```python
from build123d import *

# Parameters (mm, degrees)
CROQUIS1_W              = 30
CROQUIS1_H              = 49
SALIENTE_EXTRUIR1_DEPTH = 20
CORTAR_EXTRUIR3_DEPTH   = 20
CORTAR_EXTRUIR5_DEPTH   = 20
CORTAR_EXTRUIR6_DEPTH   = 0.3
CROQUIS5_W              = 13.233735145
CROQUIS5_H              = 2.403316153
CORTAR_EXTRUIR9_DEPTH   = 20.3
CROQUIS6_W              = 2.5
CROQUIS6_H              = 19.5
SALIENTE_EXTRUIR2_DEPTH = 29
REDONDEO1_R             = 9
CORTAR_EXTRUIR10_DEPTH  = 29
CORTAR_EXTRUIR11_DEPTH  = 29
CORTAR_EXTRUIR16_DEPTH  = 9
CORTAR_EXTRUIR17_START  = -2
CORTAR_EXTRUIR17_DEPTH  = 9
CROQUIS13_R             = 0.40141899
CORTAR_EXTRUIR18_DEPTH  = 22
MATRIZC1_COUNT          = 15
MATRIZC1_ANGLE          = 82


with BuildPart() as part:
    # Croquis1 → Saliente-Extruir1 (new body)
    with BuildSketch(Plane.XY):
        Rectangle(CROQUIS1_W, CROQUIS1_H)
    extrude(amount=SALIENTE_EXTRUIR1_DEPTH)

    # Croquis2 → Cortar-Extruir3 (cut)
    with BuildSketch(Plane.XY.offset(20)):
        with BuildLine():
            ThreePointArc((-0.474525342, 13.297985817), (-5.593414892, 15.404003131), (-9.517328589, 11.5))
            ThreePointArc((-9.517328589, 11.5), (-9.593029868, 11.00254481), (-9.618349103, 10.5))
            ThreePointArc((-9.618349103, 10.5), (-9.39256168, 9.014438062), (-8.735591395, 7.663044605))
            ThreePointArc((-8.735591395, 7.663044605), (-8.404944841, 7.234775243), (-8.029958496, 6.84474059))
            ThreePointArc((-8.029958496, 6.84474059), (-5.140673383, 3.522596276), (-3, -0.324757201))
            ThreePointArc((-3, -0.324757201), (-1.808741917, -13.286004066), (-8.416261219, -24.5))
            Line((-8.416261219, -24.5), (15, -24.5))
            Line((15, -24.5), (15, 24.5))
            Line((15, 24.5), (-8.489066238, 24.5))
            ThreePointArc((-8.489066238, 24.5), (0.804926071, 18.001388169), (2.839493239, 6.84474059))
            ThreePointArc((2.839493239, 6.84474059), (1.375466316, 10.170467938), (-0.474525342, 13.297985817))
        make_face()
    extrude(amount=-CORTAR_EXTRUIR3_DEPTH, mode=Mode.SUBTRACT)

    # Croquis3 → Cortar-Extruir5 (cut)
    with BuildSketch(Plane.XY.offset(20)):
        with BuildLine():
            Line((3.120918342, 8.787733578), (3.139240721, 10.044961504))
            ThreePointArc((3.139240721, 10.044961504), (2.537101628, 9.384743505), (1.652711167, 9.512465101))
            Line((1.652711167, 9.512465101), (2.839493239, 6.84474059))
            Line((2.839493239, 6.84474059), (3.120918342, 8.787733578))
        make_face()
    extrude(amount=-CORTAR_EXTRUIR5_DEPTH, mode=Mode.SUBTRACT)

    # Croquis4 → Cortar-Extruir6 (cut)
    with BuildSketch(Plane(origin=(2.992213613, -0.043607425, 0), x_dir=(0, 0, 1), z_dir=(-0.999893822, 0.014572086, 0))):
        Polygon((19.964912912, 10.079116377), (20.184817926, 6.981498966), (0, 6.981498966), (0, 10.089640231), align=None)
    extrude(amount=CORTAR_EXTRUIR6_DEPTH, mode=Mode.SUBTRACT)

    # Croquis5 → Cortar-Extruir9 (cut)
    with BuildSketch(Plane(origin=(2.853385744, 6.940656131, 20), x_dir=(-1, 0, 0), z_dir=(0, 0, -1))):
        with Locations((-6.558491356, -0.917958816)):
            Rectangle(CROQUIS5_W, CROQUIS5_H)
    extrude(amount=CORTAR_EXTRUIR9_DEPTH, mode=Mode.SUBTRACT)

    # Croquis6 → Saliente-Extruir2 (add)
    with BuildSketch(Plane.ZY.offset(15)):
        with Locations((16.25, -1.75)):
            Rectangle(CROQUIS6_W, CROQUIS6_H)
        with Locations((3.75, -1.75)):
            Rectangle(CROQUIS6_W, CROQUIS6_H)
    extrude(amount=SALIENTE_EXTRUIR2_DEPTH)

    # Redondeo1
    redondeo1_edges = [part.edges().sort_by_distance(p)[0] for p in [
        (-44, -11.5, 16.25),
        (-44, 8, 16.25),
        (-44, -11.5, 3.75),
        (-44, 8, 3.75),
    ]]
    fillet(redondeo1_edges, radius=REDONDEO1_R)

    # Croquis7 → Cortar-Extruir10 (cut)
    with BuildSketch(Plane(origin=(0, 0, 2.5), x_dir=(-1, 0, 0), z_dir=(0, 0, -1))):
        with BuildLine():
            Line((37.288140826, -6.5), (37.288140826, -11.204275476))
            ThreePointArc((37.288140826, -11.204275476), (38.094193196, -10.951388553), (38.872983346, -10.624038405))
            Line((38.872983346, -10.624038405), (38.872983346, 0))
            ThreePointArc((38.872983346, 0), (37.449489743, 2.16227766), (35, 3))
            Line((35, 3), (30, 3))
            Line((30, 3), (30, -6.5))
            Line((30, -6.5), (37.288140826, -6.5))
        make_face()
    extrude(amount=-CORTAR_EXTRUIR10_DEPTH, mode=Mode.SUBTRACT)

    # Croquis8 → Cortar-Extruir11 (cut)
    with BuildSketch(Plane(origin=(0, 0, 2.5), x_dir=(-1, 0, 0), z_dir=(0, 0, -1))):
        with BuildLine():
            Line((43.062257748, -6.5), (38.872983346, -6.5))
            Line((38.872983346, -6.5), (38.872983346, -10.624038405))
            ThreePointArc((38.872983346, -10.624038405), (41.313827539, -8.91370266), (43.062257748, -6.5))
        make_face()
    extrude(amount=-CORTAR_EXTRUIR11_DEPTH, mode=Mode.SUBTRACT)

    # Croquis9 → Cortar-Extruir16 (cut)
    with BuildSketch(Plane(origin=(0, 0, 0), x_dir=(-1, 0, 0), z_dir=(0, 0, -1))):
        with BuildLine():
            Line((14, -20.5), (14, 5.382636826))
            ThreePointArc((14, 5.382636826), (11.773893936, 6.335545077), (9.505438523, 5.488377807))
            ThreePointArc((9.505438523, 5.488377807), (9.450309647, 5.43520412), (9.394602253, 5.382636826))
            ThreePointArc((9.394602253, 5.382636826), (3.353377533, -7.168166886), (7.3883863, -20.5))
            ThreePointArc((7.3883863, -20.5), (7.528094247, -20.675980579), (7.669852324, -20.850313944))
            ThreePointArc((7.669852324, -20.850313944), (10.918883483, -22.192259689), (14, -20.5))
        make_face()
    extrude(amount=-CORTAR_EXTRUIR16_DEPTH, mode=Mode.SUBTRACT)

    # Croquis11 → Cortar-Extruir17 (cut)
    with BuildSketch(Plane(origin=(0, 0, 9), x_dir=(-1, 0, 0), z_dir=(0, 0, -1)).offset(CORTAR_EXTRUIR17_START)):
        with BuildLine():
            Line((14, -20.5), (14, 5.382636826))
            ThreePointArc((14, 5.382636826), (11.773893936, 6.335545077), (9.505438523, 5.488377807))
            ThreePointArc((9.505438523, 5.488377807), (9.450309647, 5.43520412), (9.394602253, 5.382636826))
            ThreePointArc((9.394602253, 5.382636826), (3.337324426, -7.392286881), (7.669852324, -20.850313944))
            ThreePointArc((7.669852324, -20.850313944), (10.918883483, -22.192259689), (14, -20.5))
        make_face()
    extrude(amount=-CORTAR_EXTRUIR17_DEPTH, mode=Mode.SUBTRACT)

    # Croquis13 → Cortar-Extruir18 (cut)
    with BuildSketch(Plane(origin=(0, 0, 0), x_dir=(-1, 0, 0), z_dir=(0, 0, -1))):
        with Locations((5.927972834, 4.573929347)):
            Circle(CROQUIS13_R)
    cortar_extruir18 = extrude(amount=-CORTAR_EXTRUIR18_DEPTH, mode=Mode.SUBTRACT)

    # MatrizC1: Cortar-Extruir18 ×15 about axis
    matrizc1_axis = Axis((-22.493499964, -8.651756801, 0), (0, 0, -1))
    for i in range(1, MATRIZC1_COUNT):
        add(cortar_extruir18.rotate(matrizc1_axis, i * MATRIZC1_ANGLE / (MATRIZC1_COUNT - 1)), mode=Mode.SUBTRACT)


solid = part.part
```
The listing builds one solid part. Answer for the finished solid, in the listing's coordinates (mm). A direction names the side the tool comes from. Give positions to 0.01 mm unless a question says otherwise; leave off trailing zeros. Order: outer loops, then holes, each group sorted by start corner. A loop starts at its lowest first (then second) coordinate and runs counter-clockwise, first axis right, second up.
1) Find section B-B on x = -27.5. Write down the section's boundary in (y, z), then the cut area to 3 significant figures.
Reported:
outline: (-11.5, 2.5) - (8, 2.5) - (8, 5) - (-11.5, 5) - close; (-11.5, 15) - (8, 15) - (8, 17.5) - (-11.5, 17.5) - close
area: 97.5 mm2
2) Consider line 1 along X through (y, z) = (0, 16); line 2 along X through (y, z) = (-19, 12); line 3 along X through (y, z) = (-8, 8). Determine where each line is inside the solid, lowest interval first.
Reported:
line 1: x = -43.94 to -38.87, -30 to -14, -5.36 to -3.14
line 2: x = -15 to -14, -6.32 to -3.99
line 3: x = -15 to -14, -3.31 to -1.31
3) Find section C-C on x = -11. Write down the section's boundary in (y, z), then the cut area to 3 significant figures.
Reported:
outline: (-24.5, 0) - (-22.19, 0) - (-22.19, 9) - (6.26, 9) - (6.26, 0) - (24.5, 0) - (24.5, 20) - (6.26, 20) - (6.26, 11) - (-22.19, 11) - (-22.19, 20) - (-24.5, 20) - close
area: 468 mm2
4) Determine the mould class of faces 4 (the face through (-4.11, 1.9, 10.14)), 5 (the face through (-25, 8, 16)), 6 (the face through (-3.35, -7.19, 15.44)), 7 (the face through (-43.756, -4.582, 16.267)) for opening direction X: pulls with the +X half, pulls with the -X half, needs draft (parallel to the pull), parting line crosses it, or undercut.
Reported:
face 4: pulls with the +X half
face 5: needs draft
face 6: undercut
face 7: pulls with the -X half
5) Find section A-A on x = -32.5. Write down the section's boundary in (y, z), then the cut area to 3 significant figures.
Reported:
outline: (-11.5, 2.5) - (-6.5, 2.5) - (-6.5, 5) - (-11.5, 5) - close; (-11.5, 15) - (-6.5, 15) - (-6.5, 17.5) - (-11.5, 17.5) - close; (3, 2.5) - (8, 2.5) - (8, 5) - (3, 5) - close; (3, 15) - (8, 15) - (8, 17.5) - (3, 17.5) - close
area: 50.0 mm2
6) Given P1, Ø0.8, axis at x = -21.5, z = 16.5, coming from the +Y side; P2, Ø5.5, axis at x = -10.5, y = -13, coming from the -Z side; P3, Ø0.8, axis at y = -3.5, z = 4, coming from the +X side; P4, Ø10, axis at x = -36.5, y = -18.5, coming from the +Z side, each flat-ended and moving along its own axis, determine where each tip first touches the part or whether it passes through.
Reported:
P1: stops at y = 8
P2: stops at z = 9
P3: stops at x = -1.84
P4: passes through
7) Find section D-D on x = -40. Write down the section's boundary in (y, z), then the cut area to 3 significant figures.
Reported:
outline: (-6.5, 2.5) - (6.48, 2.5) - (6.48, 5) - (-6.5, 5) - close; (-6.5, 15) - (6.48, 15) - (6.48, 17.5) - (-6.5, 17.5) - close
area: 64.9 mm2
8) For faces 1 (the face through (-25, -11.5, 4)), 2 (the face through (-26, -2, 5)), 3 (the face through (-37.48, 2.14, 3.73)), determine the directions among +Z, -Z, +X, -X, +Y, -Y from which every point of the face is accessible in a straight line to the end or side of a thin tool.
Reported:
face 1: +Z, -Z, -X, -Y
face 2: -X, +Y, -Y
face 3: +Z, -Z
